Design review of the part built by this model. Coordinates are the model's own, in mm. A direction names the side the tool comes from. Coordinates: 2 decimals unless noted, no trailing zeros. Loops run counter-clockwise (first coordinate to the right, second up) from the corner with the lowest first, then second, coordinate; pieces in that order, holes last. Notation, with made-up numbers: (28, -17.5) - (35, -17.5) arc R22 ccw to (35, -4.5) - close; hole circle Ø9 at (87, 24.25). An arc over 180 degrees is marked (long way). One line per question, with ' | ' between items.
from build123d import *

# Parameters (mm, degrees)
F1_DEPTH     = 12.7
F2_DEPTH     = 25.4
F3_DEPTH     = 63.5
F4_R         = 6.34999
F5_T1_DEPTH  = 103.9650864339
F5_T3_DEPTH  = 58.332543217
F5_T5_DEPTH  = 58.332543217
F5_T7_DEPTH  = 103.9650864339
F5_T9_DEPTH  = 103.9650864339
F5_T11_DEPTH = 103.9650864339
F5_T13_DEPTH = 58.332543217
F5_T15_DEPTH = 58.332543217
F5_T18_ANGLE = 90
F5_T20_ANGLE = 90


# Not quite as in the source:
# - a fillet or chamfer that OpenCascade refuses, or shapes differently, is made with other operations: its cross-section is extruded or revolved along the edge and cut away or added
# - a fillet or chamfer is up to 0.001 mm smaller than in the source, because OpenCascade refuses the exact size
# - a feature of the source that left no trace in its solid (it failed there, or was rolled back) is left out


with BuildPart() as f1:
    # F0 (on Top) → F1 (new body)
    with BuildSketch(Plane.XY):
        Polygon((38.0595053568, 82.2464972734), (-38.0927510742, 82.2464972734), (-44.45, 82.2464972734), (-44.45, 76.2), (-44.45, -82.8535027266), (-38.1, -82.8535027266), (44.45, -82.8535027266), (44.45, 82.2464972734), align=None)
        Polygon((-38.1, -76.5035027266), (-38.1, 0), (-38.1, 37.7964972734), (-38.1, 75.8964972734), (0, 75.8964972734), (38.1, 75.8964972734), (38.1, -38.4035027266), (38.1, -76.5035027266), (0, -76.5035027266), align=None, mode=Mode.SUBTRACT)
        with BuildLine():
            Line((-38.1, 75.8964972734), (-38.1, 37.7964972734))
            Line((-38.1, 37.7964972734), (-12.7, 37.7964972734))
            ThreePointArc((-12.7, 37.7964972734), (-3.7197438789, 41.5162411524), (0, 50.4964972734))
            Line((0, 50.4964972734), (0, 75.8964972734))
            Line((0, 75.8964972734), (-38.1, 75.8964972734))
        make_face()
        with BuildLine():
            Line((-38.1, 37.7964972734), (-38.1, 0))
            Line((-38.1, 0), (-38.1, -76.5035027266))
            Line((-38.1, -76.5035027266), (0, -76.5035027266))
            Line((0, -76.5035027266), (0, -51.1035027266))
            ThreePointArc((0, -51.1035027266), (3.7197438789, -42.1232466055), (12.7, -38.4035027266))
            Line((12.7, -38.4035027266), (38.1, -38.4035027266))
            Line((38.1, -38.4035027266), (38.1, 75.8964972734))
            Line((38.1, 75.8964972734), (0, 75.8964972734))
            Line((0, 75.8964972734), (0, 50.4964972734))
            ThreePointArc((0, 50.4964972734), (-3.7197438789, 41.5162411524), (-12.7, 37.7964972734))
            Line((-12.7, 37.7964972734), (-38.1, 37.7964972734))
        make_face()
        with BuildLine():
            Line((0, -51.1035027266), (0, -76.5035027266))
            Line((0, -76.5035027266), (38.1, -76.5035027266))
            Line((38.1, -76.5035027266), (38.1, -38.4035027266))
            Line((38.1, -38.4035027266), (12.7, -38.4035027266))
            ThreePointArc((12.7, -38.4035027266), (3.7197438789, -42.1232466055), (0, -51.1035027266))
        make_face()
    extrude(amount=F1_DEPTH)

    # F0 (on Top) → F2 (join)
    with BuildSketch(Plane.XY):
        with BuildLine():
            Line((0, -51.1035027266), (0, -76.5035027266))
            Line((0, -76.5035027266), (38.1, -76.5035027266))
            Line((38.1, -76.5035027266), (38.1, -38.4035027266))
            Line((38.1, -38.4035027266), (12.7, -38.4035027266))
            ThreePointArc((12.7, -38.4035027266), (3.7197438789, -42.1232466055), (0, -51.1035027266))
        make_face()
        with BuildLine():
            Line((-38.1, 37.7964972734), (-38.1, 0))
            Line((-38.1, 0), (-38.1, -76.5035027266))
            Line((-38.1, -76.5035027266), (0, -76.5035027266))
            Line((0, -76.5035027266), (0, -51.1035027266))
            ThreePointArc((0, -51.1035027266), (3.7197438789, -42.1232466055), (12.7, -38.4035027266))
            Line((12.7, -38.4035027266), (38.1, -38.4035027266))
            Line((38.1, -38.4035027266), (38.1, 75.8964972734))
            Line((38.1, 75.8964972734), (0, 75.8964972734))
            Line((0, 75.8964972734), (0, 50.4964972734))
            ThreePointArc((0, 50.4964972734), (-3.7197438789, 41.5162411524), (-12.7, 37.7964972734))
            Line((-12.7, 37.7964972734), (-38.1, 37.7964972734))
        make_face()
        with BuildLine():
            Line((-38.1, 75.8964972734), (-38.1, 37.7964972734))
            Line((-38.1, 37.7964972734), (-12.7, 37.7964972734))
            ThreePointArc((-12.7, 37.7964972734), (-3.7197438789, 41.5162411524), (0, 50.4964972734))
            Line((0, 50.4964972734), (0, 75.8964972734))
            Line((0, 75.8964972734), (-38.1, 75.8964972734))
        make_face()
    extrude(amount=F2_DEPTH)

    # F0 (on Top) → F3 (join)
    with BuildSketch(Plane.XY):
        with BuildLine():
            Line((0, -51.1035027266), (0, -76.5035027266))
            Line((0, -76.5035027266), (38.1, -76.5035027266))
            Line((38.1, -76.5035027266), (38.1, -38.4035027266))
            Line((38.1, -38.4035027266), (12.7, -38.4035027266))
            ThreePointArc((12.7, -38.4035027266), (3.7197438789, -42.1232466055), (0, -51.1035027266))
        make_face()
        with BuildLine():
            Line((-38.1, 75.8964972734), (-38.1, 37.7964972734))
            Line((-38.1, 37.7964972734), (-12.7, 37.7964972734))
            ThreePointArc((-12.7, 37.7964972734), (-3.7197438789, 41.5162411524), (0, 50.4964972734))
            Line((0, 50.4964972734), (0, 75.8964972734))
            Line((0, 75.8964972734), (-38.1, 75.8964972734))
        make_face()
    extrude(amount=F3_DEPTH)

    # F4 (radius 6.35 in the source; OpenCascade refuses exactly that, so slightly less here)
    f4_edges = [f1.edges().sort_by_distance(p)[0] for p in [
        (-44.45, -0.303503, 12.7),
        (0, -82.853503, 12.7),
        (44.45, -0.303503, 12.7),
        (0, 82.246497, 12.7),
    ]]
    fillet(f4_edges, radius=F4_R)

    # F5: chamfer of 5.08 x 12.7 on 10 edges, made by hand

    # F5_s2 → F5_t1 (cut)
    with BuildSketch(Plane.XZ.offset(5.4709595096)):
        Polygon((38.1, 50.8), (33.02, 63.5), (38.1, 63.5), align=None)
    extrude(amount=F5_T1_DEPTH, mode=Mode.SUBTRACT)

    # F5_s4 → F5_t3 (cut)
    with BuildSketch(Plane.YZ.offset(12.7)):
        Polygon((-43.4835027266, 63.5), (-38.4035027266, 50.8), (-38.4035027266, 63.5), align=None)
    extrude(amount=F5_T3_DEPTH, mode=Mode.SUBTRACT)

    # F5_s6 → F5_t5 (cut)
    with BuildSketch(Plane.XZ.offset(51.1035027266)):
        Polygon((5.08, 63.5), (0, 50.8), (0, 63.5), align=None)
    extrude(amount=F5_T5_DEPTH, mode=Mode.SUBTRACT)

    # F5_s8 → F5_t7 (cut)
    with BuildSketch(Plane.YZ.offset(-32.932543217)):
        Polygon((-76.5035027266, 50.8), (-71.4235027266, 63.5), (-76.5035027266, 63.5), align=None)
    extrude(amount=F5_T7_DEPTH, mode=Mode.SUBTRACT)

    # F5_s10 → F5_t9 (cut)
    with BuildSketch(Plane.YZ.offset(-71.032543217)):
        Polygon((75.8964972734, 50.8), (70.8164972734, 63.5), (75.8964972734, 63.5), align=None)
    extrude(amount=F5_T9_DEPTH, mode=Mode.SUBTRACT)

    # F5_s12 → F5_t11 (cut)
    with BuildSketch(Plane.XZ.offset(-108.8290404904)):
        Polygon((-38.1, 50.8), (-33.02, 63.5), (-38.1, 63.5), align=None)
    extrude(amount=F5_T11_DEPTH, mode=Mode.SUBTRACT)

    # F5_s14 → F5_t13 (cut)
    with BuildSketch(Plane.XZ.offset(-108.8290404904)):
        Polygon((0, 50.8), (-5.08, 63.5), (0, 63.5), align=None)
    extrude(amount=F5_T13_DEPTH, mode=Mode.SUBTRACT)

    # F5_s16 → F5_t15 (cut)
    with BuildSketch(Plane.YZ.offset(-71.032543217)):
        Polygon((42.8764972734, 63.5), (37.7964972734, 50.8), (37.7964972734, 63.5), align=None)
    extrude(amount=F5_T15_DEPTH, mode=Mode.SUBTRACT)

    # F5_s17 → F5_t18 (revolve, cut)
    with BuildSketch(Plane.YZ.offset(12.7)):
        Polygon((-43.4835027266, 63.5), (-38.4035027266, 50.8), (-38.4035027266, 63.5), align=None)
    revolve(axis=Axis((12.7, -51.1035027266, 63.5), (0, 0, 1)), revolution_arc=F5_T18_ANGLE, mode=Mode.SUBTRACT)

    # F5_s19 → F5_t20 (revolve, cut)
    with BuildSketch(Plane.YZ.offset(-12.7)):
        Polygon((42.8764972734, 63.5), (37.7964972734, 50.8), (37.7964972734, 63.5), align=None)
    revolve(axis=Axis((-12.7, 50.4964972734, 63.5), (0, 0, 1)), revolution_arc=F5_T20_ANGLE, mode=Mode.SUBTRACT)


solid = f1.part
Q1. To check wall thickness, follow line 1 along X through (y, z) = (-58, 14.5); line 2 along Y through (x, z) = (-28, 30); line 3 along Z through (x, y) = (24, 58.5). State the ranges of each line that lie inside material, in increasing order.
Returned:
line 1: x = -38.1 to 38.1 | line 2: y = 37.8 to 75.9 | line 3: z = 0 to 25.4
Q2. Tool access review of faces 1 (the flat face through (-38.1, 18, 23)), 2 (the flat face through (8, -76.504, 27)), 3 (the flat face through (0, 63, 38)), 4 (the flat face through (26, -38.404, 38)): name each direction out of +Z, -Z, +X, -X, +Y, -Y from which nothing blocks a thin tool from reaching the whole face with its end or side.
Returned:
face 1: +Z, -X, +Y, -Y | face 2: +Z, +X, -X, -Y | face 3: +Z, +X, +Y | face 4: +Z, +X, -X, +Y
Q3. Take a section at A-A (z = 30). Give the boundary of the cut face in (x, y).
Returned:
outline: (-38.1, 37.8) - (-12.7, 37.8) arc R12.7 ccw to (0, 50.5) - (0, 75.9) - (-38.1, 75.9) - close; (0, -76.5) - (38.1, -76.5) - (38.1, -38.4) - (12.7, -38.4) arc R12.7 ccw to (0, -51.1) - close
Q4. For pin 1 (7.5 mm diameter, centred on x = -19.5, z = 38, fed in from -Y); pin 2 (10 mm diameter, centred on x = 32.5, z = 42.5, fed in from +Y); pin 3 (3 mm diameter, centred on x = 34, z = 18.5, fed in from -Y), all flat-tipped, find the tip position at first contact; note any pin that passes through.
Returned:
pin 1: stops at y = 37.8 | pin 2: stops at y = -38.4 | pin 3: stops at y = -76.5
